Geometry: final body of the model. Coordinates: model frame, mm. Face numbers are marked on the shaded views. A direction names the side the tool comes from. Round coordinates to 2 decimals unless told otherwise and drop trailing zeros. Write each loop counter-clockwise with the first axis right and the second up, starting at its lowest first coordinate (ties: lowest second). Pieces come first, ordered by that corner, then holes. Notation, with made-up numbers: (59, 51) -> (78, 51) arc R24 cw to (78, 72) -> close; hole circle Ø3 at (-14.5, 58.5). An arc over 180 degrees is marked (long way). One line per item, written item: value. Start each with the question number.
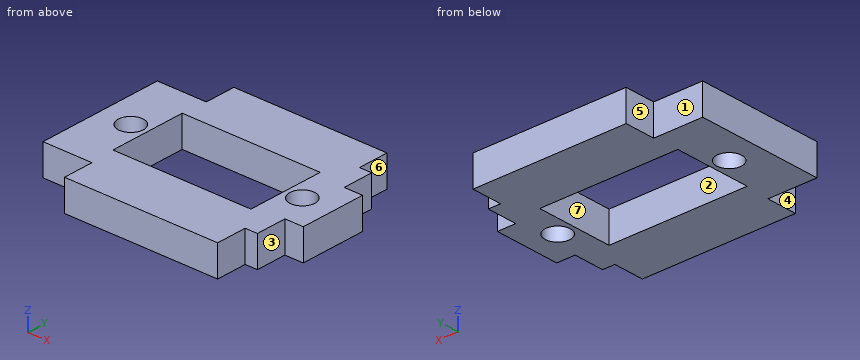
from build123d import *

# Parameters (mm, degrees)
SALIENTE_EXTRUIR1_DEPTH = 5
CUT_EXTRUDE1_REACH      = 7
CROQUIS2_R              = 2.05
CROQUIS2_W              = 22.53
CROQUIS2_H              = 12.6


with BuildPart() as part:
    # Croquis1 → Saliente-Extruir1 (new body)
    with BuildSketch(Plane.XY):
        Polygon((-12.5, 15.39), (12.5, 15.39), (12.5, 10.39), (14.5, 10.39), (14.5, 5.39), (17.5, 5.39), (17.5, -5.39), (14.5, -5.39), (14.5, -10.39), (12.5, -10.39), (12.5, -15.39), (-12.5, -15.39), (-12.5, -10.39), (-20.5, -10.39), (-20.5, 10.39), (-12.5, 10.39), align=None)
    extrude(amount=SALIENTE_EXTRUIR1_DEPTH)

    # Croquis2 → Cut-Extrude1 (cut, up to next)
    with BuildSketch(Plane.XY.offset(5), mode=Mode.PRIVATE) as cut_extrude1_sk1:
        with Locations((-15.5, 0)):
            Circle(CROQUIS2_R)
    cut_extrude1_tool1 = extrude(cut_extrude1_sk1.sketch, amount=-CUT_EXTRUDE1_REACH, mode=Mode.PRIVATE) & part.part
    add(cut_extrude1_tool1.solids().sort_by_distance((-15.5, 0, 5))[0], mode=Mode.SUBTRACT)
    # Croquis2 → Cut-Extrude1 (cut, up to next)
    with BuildSketch(Plane.XY.offset(5), mode=Mode.PRIVATE) as cut_extrude1_sk2:
        with Locations((12.5035, 0)):
            Circle(CROQUIS2_R)
    cut_extrude1_tool2 = extrude(cut_extrude1_sk2.sketch, amount=-CUT_EXTRUDE1_REACH, mode=Mode.PRIVATE) & part.part
    add(cut_extrude1_tool2.solids().sort_by_distance((12.5035, 0, 5))[0], mode=Mode.SUBTRACT)
    # Croquis2 → Cut-Extrude1 (cut, up to next)
    with BuildSketch(Plane.XY.offset(5), mode=Mode.PRIVATE) as cut_extrude1_sk3:
        with Locations((-1.49835, 0)):
            Rectangle(CROQUIS2_W, CROQUIS2_H)
    cut_extrude1_tool3 = extrude(cut_extrude1_sk3.sketch, amount=-CUT_EXTRUDE1_REACH, mode=Mode.PRIVATE) & part.part
    add(cut_extrude1_tool3.solids().sort_by_distance((-1.49835, 0, 5))[0], mode=Mode.SUBTRACT)


solid = part.part
(1) Line query: probe 1 along Y at (x, z) = (-8.5, 1.55); probe 2 along X at (y, z) = (-1, 1.95); probe 3 along X at (y, z) = (0.5, 3.35). Output: solid intervals per line, ascending.
(2) Section query D-D (x = -15.5). Output: boundary loops of the cut face in (y, z), and give its area (3 significant figures).
(3) Section query C-C (z = 2.75). Output: boundary loops of the cut face in (x, y), and give its area (3 significant figures).
(4) Pin query (flat end, axial travel): pin 1 (2.5 mm diameter, centred on x = 15.5, z = 2, fed in from +Y); pin 2 (2.5 mm diameter, centred on y = 13.5, z = 2, fed in from +X); pin 3 (1.5 mm diameter, centred on y = 8, z = 1.5, fed in from +X). Return the tip coordinate at first contact, or that it passes through.
(5) Pull-direction query (X, two-part tool) for the marked faces 1, 2 and 3; classes: pulls with the +X half, pulls with the -X half, needs draft (parallel to the pull), parting line crosses it, or undercut.
(6) Section query B-B (x = -10.5). Output: boundary loops of the cut face in (y, z).
(7) Section query A-A (y = 0). Output: boundary loops of the cut face in (x, z).
(8) Set-up query: the marked faces 4, 5, 6 and 7. Return all of +Z, -Z, +X, -X, +Y, -Y with unobstructed straight access to the full face (end or side cutting, diameter ignored); none if empty.
Results list:
1. probe 1: y = -15.39 to -6.3, 6.3 to 15.39
1. probe 2: x = -20.5 to -17.29, -13.71 to -12.76, 9.77 to 10.71, 14.29 to 17.5
1. probe 3: x = -20.5 to -17.49, -13.51 to -12.76, 9.77 to 10.52, 14.49 to 17.5
2. outline: (-10.39, 0) -> (-2.05, 0) -> (-2.05, 5) -> (-10.39, 5) -> close; (2.05, 0) -> (10.39, 0) -> (10.39, 5) -> (2.05, 5) -> close
2. area: 83.4 mm^2
3. outline: (-20.5, -10.39) -> (-12.5, -10.39) -> (-12.5, -15.39) -> (12.5, -15.39) -> (12.5, -10.39) -> (14.5, -10.39) -> (14.5, -5.39) -> (17.5, -5.39) -> (17.5, 5.39) -> (14.5, 5.39) -> (14.5, 10.39) -> (12.5, 10.39) -> (12.5, 15.39) -> (-12.5, 15.39) -> (-12.5, 10.39) -> (-20.5, 10.39) -> close; hole circle Ø4.1 at (-15.5, 0); hole (-12.76, -6.3) -> (9.77, -6.3) -> (9.77, 6.3) -> (-12.76, 6.3) -> close; hole circle Ø4.1 at (12.5, 0)
3. area: 699 mm^2
4. pin 1: stops at y = 10.39
4. pin 2: stops at x = 12.5
4. pin 3: stops at x = 14.5
5. face 1: needs draft
5. face 2: undercut
5. face 3: pulls with the +X half
6. outline: (-15.39, 0) -> (-6.3, 0) -> (-6.3, 5) -> (-15.39, 5) -> close; (6.3, 0) -> (15.39, 0) -> (15.39, 5) -> (6.3, 5) -> close
7. outline: (-20.5, 0) -> (-17.55, 0) -> (-17.55, 5) -> (-20.5, 5) -> close; (-13.45, 0) -> (-12.76, 0) -> (-12.76, 5) -> (-13.45, 5) -> close; (9.77, 0) -> (10.45, 0) -> (10.45, 5) -> (9.77, 5) -> close; (14.55, 0) -> (17.5, 0) -> (17.5, 5) -> (14.55, 5) -> close
8. face 4: +Z, -Z, -X, -Y
8. face 5: +Z, -Z, -X, +Y
8. face 6: +Z, -Z, +X, +Y
8. face 7: +Z, -Z
